Design review of the part built by this model. Coordinates are the model's own, in mm. A direction names the side the tool comes from. Coordinates: 2 decimals unless noted, no trailing zeros. Write each loop counter-clockwise with the first axis right and the second up, starting at its lowest first coordinate (ties: lowest second). Pieces come first, ordered by that corner, then holes. Notation, with made-up numbers: (23.25, -17) -> (27.25, -17) arc R21 ccw to (27.25, 2) -> close; hole circle Ø9 at (42, -25.5). An arc over 180 degrees is marked (long way). Answer in a Markdown table with one row per item. Add a question column.
Item 1: Take a section at B-B, the plane z = -400. Write out the cut boundary in (x, y), and give its area (3 significant figures).
Item 2: To check wall thickness, follow line 1 (X direction, y = 8.5, z = -400); line 2 (Z direction, x = 89, y = 68); line 3 (X direction, y = 58, z = -214.5). State the ranges of each line that lie inside material, in increasing order.
Item 3: Clearance check with flat-ended pins moving along their axes: P1, Ø9.5, axis at x = 137.5, z = -365.5, coming from the +Y side; P2, Ø22.5, axis at y = 54, z = -167, coming from the +X side; P3, Ø1.5, axis at x = 202.5, y = 43, coming from the -Z side. State where each tip first meets the part, or that it passes through.
Item 4: Draft analysis for pull direction X (two halves, no side actions). For faces 1 (the face through (348.8, 81, -224.9)), 2 (the face through (98.775, 79.113, -99.916)), 3 (the face through (143.5, 49, -162)), state which applies: released by +X, released by -X, zero draft, split by the parting line, or undercut.
Item 5: Take a section at C-C, the plane y = 104.5. Write out the cut boundary in (x, z).
Item 6: Take a section at A-A, the plane x = 225. Give the number of separate pieces and of enclosed holes in the cut face, and give its area (3 significant figures).
Item 7: Take a section at D-D, the plane z = -100. Write out the cut boundary in (x, y).
Item 8: For faces 4 (the face through (306.5, 41, -67)), 5 (the face through (225, 87, -365)), 6 (the face through (225, 62, -162)), 7 (the face through (131.5, 49, -162)), list the 3-axis set-ups (+Z, -Z, +X, -X, +Y, -Y) from which the entire face can be reached by the end or side of a thin tool; tool diameter is ignored.
from build123d import *

# Parameters (mm, degrees)
SKETCH_1_W          = 450
SKETCH_1_H          = 450
EXTRUDE_1_DEPTH     = 12
SKETCH_2_R          = 11.5
CUT_EXTRUDE_1_DEPTH = 637.509230098
SKETCH_5_W          = 450
SKETCH_5_H          = 12
EXTRUDE_2_DEPTH     = 150
SKETCH_6_R          = 25
CUT_EXTRUDE_2_DEPTH = 597.221435374
SKETCH_7_W          = 12
SKETCH_7_H          = 75
EXTRUDE_3_DEPTH     = 450
CUT_EXTRUDE_4_DEPTH = 575.337226723
SKETCH_10_W         = 113
SKETCH_10_H         = 25
CUT_EXTRUDE_5_DEPTH = 12


with BuildPart() as part:
    # 草图1 → 凸台-拉伸1 (new body)
    with BuildSketch(Plane(origin=(0, 0, 0), x_dir=(1, 0, 0), z_dir=(0, 1, 0))):
        with Locations((225, 225)):
            Rectangle(SKETCH_1_W, SKETCH_1_H)
    extrude(amount=EXTRUDE_1_DEPTH)

    # 草图2 → 切除-拉伸1 (cut, through all)
    with BuildSketch(Plane(origin=(0, 12, 0), x_dir=(1, 0, 0), z_dir=(0, 1, 0))):
        with Locations(Location((100, 50, 0), (0, 0, 270))):
            Circle(SKETCH_2_R)
        with Locations(Location((100, 400, 0), (0, 0, 270))):
            Circle(SKETCH_2_R)
        with Locations(Location((350, 400, 0), (0, 0, 270))):
            Circle(SKETCH_2_R)
        with Locations(Location((350, 50, 0), (0, 0, 270))):
            Circle(SKETCH_2_R)
    extrude(amount=-CUT_EXTRUDE_1_DEPTH, mode=Mode.SUBTRACT)

    # 草图5 → 凸台-拉伸2 (add)
    with BuildSketch(Plane(origin=(0, 12, 0), x_dir=(1, 0, 0), z_dir=(0, 1, 0))):
        with Locations((225, 350)):
            Rectangle(SKETCH_5_W, SKETCH_5_H)
        with Locations((225, 225)):
            Rectangle(SKETCH_5_W, SKETCH_5_H)
        with Locations((225, 100)):
            Rectangle(SKETCH_5_W, SKETCH_5_H)
    extrude(amount=EXTRUDE_2_DEPTH)

    # 草图6 → 切除-拉伸2 (cut, through all)
    with BuildSketch(Plane.XY.offset(-94)):
        with Locations((225, 120)):
            Circle(SKETCH_6_R)
        with BuildLine():
            Line((0, 162), (0, 12))
            Line((0, 12), (12.5, 12))
            Line((12.5, 12), (187.5, 148.131907659))
            ThreePointArc((187.5, 148.131907659), (225, 161), (262.5, 148.131907659))
            Line((262.5, 148.131907659), (437.5, 12))
            Line((437.5, 12), (450, 12))
            Line((450, 12), (450, 162))
            Line((450, 162), (0, 162))
        make_face()
    extrude(amount=-CUT_EXTRUDE_2_DEPTH, mode=Mode.SUBTRACT)

    # 草图7 → 凸台-拉伸3 (add)
    with BuildSketch(Plane.XY):
        with Locations((225, 49.5)):
            Rectangle(SKETCH_7_W, SKETCH_7_H)
        with Locations((137.5, 49.5)):
            Rectangle(SKETCH_7_W, SKETCH_7_H)
        with Locations((312.5, 49.5)):
            Rectangle(SKETCH_7_W, SKETCH_7_H)
    extrude(amount=-EXTRUDE_3_DEPTH)

    # 草图9 → 切除-拉伸4 (cut, through all)
    with BuildSketch(Plane.ZY.offset(-131.5)):
        Polygon((-450, 87), (-375, 87), (-425, 12), (-450, 12), align=None)
        Polygon((0, 87), (-75, 87), (-25, 12), (0, 12), align=None)
    extrude(amount=-CUT_EXTRUDE_4_DEPTH, mode=Mode.SUBTRACT)

    # 草图10 → 切除-拉伸5 (cut)
    with BuildSketch(Plane(origin=(231, 0, 0), x_dir=(0, 0, -1), z_dir=(1, 0, 0))):
        with Locations((162.5, 74.5)):
            Rectangle(SKETCH_10_W, SKETCH_10_H)
        with Locations((287.5, 74.5)):
            Rectangle(SKETCH_10_W, SKETCH_10_H)
    extrude(amount=-CUT_EXTRUDE_5_DEPTH, mode=Mode.SUBTRACT)


solid = part.part
Answers:
| question | item | result |
|---|---|---|
| 1 | outline | (0, 0) -> (88.5, 0) -> (88.5, 12) -> (0, 12) -> close; (111.5, 0) -> (338.5, 0) -> (338.5, 12) -> (318.5, 12) -> (318.5, 49.5) -> (306.5, 49.5) -> (306.5, 12) -> (231, 12) -> (231, 49.5) -> (219, 49.5) -> (219, 12) -> (143.5, 12) -> (143.5, 49.5) -> (131.5, 49.5) -> (131.5, 12) -> (111.5, 12) -> close; (361.5, 0) -> (450, 0) -> (450, 12) -> (361.5, 12) -> close |
| 1 | area | 6,200 mm^2 |
| 2 | line 1 | x = 0 to 88.5, 111.5 to 338.5, 361.5 to 450 |
| 2 | line 2 | z = -356 to -344, -231 to -219, -106 to -94 |
| 2 | line 3 | x = 131.5 to 143.5, 219 to 231, 306.5 to 318.5 |
| 3 | P1 | stops at y = 87 |
| 3 | P2 | stops at x = 318.5 |
| 3 | P3 | stops at z = -356 |
| 4 | face 1 | released by +X |
| 4 | face 2 | released by -X |
| 4 | face 3 | undercut |
| 5 | outline | (131.41, -356) -> (205.38, -356) -> (205.38, -344) -> (131.41, -344) -> close; (131.41, -231) -> (205.38, -231) -> (205.38, -219) -> (131.41, -219) -> close; (131.41, -106) -> (205.38, -106) -> (205.38, -94) -> (131.41, -94) -> close; (244.62, -356) -> (318.59, -356) -> (318.59, -344) -> (244.62, -344) -> close; (244.62, -231) -> (318.59, -231) -> (318.59, -219) -> (244.62, -219) -> close; (244.62, -106) -> (318.59, -106) -> (318.59, -94) -> (244.62, -94) -> close |
| 6 | separate pieces | 4 |
| 6 | enclosed holes | 0 |
| 6 | area | 26,900 mm^2 |
| 7 | outline | (0, 0) -> (450, 0) -> (450, 12) -> (437.5, 12) -> (262.5, 148.13) arc R61.08 ccw to (187.5, 148.13) -> (12.5, 12) -> (0, 12) -> close; hole circle Ø50 at (225, 120) |
| 8 | face 4 | +Z, +Y |
| 8 | face 5 | -Z, +X, -X, +Y |
| 8 | face 6 | +Y |
| 8 | face 7 | -X, +Y |
